Could you check a few things on this model? Use its own coordinates, in mm. Round coordinates to 2 decimals unless told otherwise and drop trailing zeros. Write each loop counter-clockwise with the first axis right and the second up, starting at its lowest first coordinate (ties: lowest second). Pieces come first, ordered by that corner, then holes. Notation, with made-up numbers: M 80,6 L 136,6 A12 cw 136,19 Z; hole C 29.25,10 d9. An arc over 180 degrees is marked long. One line per item, written item: value. Start each with the question number.
(1) If I drill on L1, parallel to Y at x = 0, z = 2.05; L2, parallel to Y at x = -17, z = 1.7, over which ranges is the centre line in solid material (lowest first)?
(2) I'm going to push flat-ended pins straight in: pin 1 Ø2 at (y, z) = (-199.5, 2.5) entering from -X; pin 2 Ø2 at (y, z) = (-200.5, 1) entering from +X; pin 3 Ø1.2 at (x, z) = (200.5, 1) entering from -Y. Where does each tip first touch, or does it pass through?
(3) I want a section at A-A on y = -142. Please give me the cut outline in (x, z).
(4) I want a section at B-B on x = 0. Please give me the cut outline in (y, z).
(5) Thinking about a two-plate mould opening in Y: for faces 1 (the face through (-0.976, -134.564, 2.028)), 2 (the face through (-3, 3, 0)), which applies, released by +Y, released by -Y, zero draft, split by the parting line, or undercut?
```python
from build123d import *

# Parameters (mm, degrees)
SKETCH1_W           = 419
SKETCH1_H           = 419
BASE_SHEET_DEPTH    = 4
SKETCH2_W           = 19.5
SKETCH2_H           = 34.5
BELT_CUTOUTS_DEPTH  = 297.304741778
SKETCH3_R           = 7.5
SKETCH3_W           = 40
SKETCH3_H           = 25
CABLE_CUTOUTS_DEPTH = 4
FILLET1_R           = 3


with BuildPart() as part:
    # Sketch1 → base sheet (new body)
    with BuildSketch(Plane.XY):
        Rectangle(SKETCH1_W, SKETCH1_H)
    extrude(amount=BASE_SHEET_DEPTH)

    # Sketch2 → belt cutouts (cut, through all)
    with BuildSketch(Plane.XY.offset(4)):
        with Locations((-199.75, 192.25)):
            Rectangle(SKETCH2_W, SKETCH2_H)
        with Locations((199.75, 192.25)):
            Rectangle(SKETCH2_W, SKETCH2_H)
        with Locations((-199.75, -192.25)):
            Rectangle(SKETCH2_W, SKETCH2_H)
        with Locations((199.75, -192.25)):
            Rectangle(SKETCH2_W, SKETCH2_H)
    extrude(amount=-BELT_CUTOUTS_DEPTH, mode=Mode.SUBTRACT)

    # Sketch3 → cable cutouts (cut)
    with BuildSketch(Plane.XY.offset(4)):
        with Locations((0, -142)):
            Circle(SKETCH3_R)
        with Locations((0, -197)):
            Rectangle(SKETCH3_W, SKETCH3_H)
    extrude(amount=-CABLE_CUTOUTS_DEPTH, mode=Mode.SUBTRACT)

    # Fillet1
    fillet1_edges = [part.edges().sort_by_distance(p)[0] for p in [
        (209.5, 175, 2),
        (190, 175, 2),
        (190, 209.5, 2),
        (-209.5, -175, 2),
        (-190, -175, 2),
        (-190, -209.5, 2),
        (209.5, -175, 2),
        (190, -209.5, 2),
        (190, -175, 2),
        (-209.5, 175, 2),
        (-190, 209.5, 2),
        (-190, 175, 2),
        (-20, -209.5, 2),
        (-20, -184.5, 2),
        (20, -184.5, 2),
        (20, -209.5, 2),
    ]]
    fillet(fillet1_edges, radius=FILLET1_R)


solid = part.part
```
Found:
1. L1: y = -184.5 to -149.5, -134.5 to 209.5
1. L2: y = -184.5 to 209.5
2. pin 1: stops at x = -190
2. pin 2: stops at x = 190
2. pin 3: stops at y = -175
3. outline: M -209.5,0 L -7.5,0 L -7.5,4 L -209.5,4 Z; M 7.5,0 L 209.5,0 L 209.5,4 L 7.5,4 Z
4. outline: M -184.5,0 L -149.5,0 L -149.5,4 L -184.5,4 Z; M -134.5,0 L 209.5,0 L 209.5,4 L -134.5,4 Z
5. face 1: undercut
5. face 2: zero draft
